```python
from build123d import *

# Parameters (mm, degrees)
SKETCH_1_W             = 42
SKETCH_1_H             = 45
SKETCH_1_R             = 12.5
EXTRUDE_1_DEPTH        = 35
SKETCH_3_W             = 24
SKETCH_3_H             = 37
CUT_EXTRUDE_1_DEPTH    = 71.809603868
HOLE_WIZARD_M3_2_D     = 2.5
HOLE_WIZARD_M3_2_DEPTH = 6
HOLE_WIZARD_M3_2_TIP   = 0.751075774
HOLE_WIZARD_M3_4_D     = 2.5
HOLE_WIZARD_M3_4_DEPTH = 6
HOLE_WIZARD_M3_4_TIP   = 0.751075774
SKETCH_18_W            = 28
SKETCH_18_H            = 20
CUT_EXTRUDE_8_DEPTH    = 71.809603868
SKETCH_13_R            = 2
CUT_EXTRUDE_10_DEPTH   = 71.809603868
FILLET_3_DEPTH         = 42
FILLET_7_R             = 2
CUT_EXTRUDE_9_REACH    = 72.81
SKETCH_12_R            = 13
SKETCH_12_R_2          = 12.5
SKETCH_12_R_3          = 2.5


with BuildPart() as part:
    # 草图1 → 凸台-拉伸1 (new body)
    with BuildSketch(Plane.XY):
        with Locations((21, 22.5)):
            Rectangle(SKETCH_1_W, SKETCH_1_H)
        with Locations((21, 22.5)):
            Circle(SKETCH_1_R, mode=Mode.SUBTRACT)
    extrude(amount=EXTRUDE_1_DEPTH)

    # 草图3 → 切除-拉伸1 (cut, through all)
    with BuildSketch(Plane.ZY):
        with Locations((20, 22.5)):
            Rectangle(SKETCH_3_W, SKETCH_3_H)
    extrude(amount=-CUT_EXTRUDE_1_DEPTH, mode=Mode.SUBTRACT)

    # M3 螺纹孔2
    with Locations(Plane(origin=(3.5, 45, 5), x_dir=(0, 0, 1), z_dir=(0, 1, 0))):
        with Locations((0, 0), (0, 35), (22, 35), (22, 0)):
            Hole(HOLE_WIZARD_M3_2_D / 2, depth=HOLE_WIZARD_M3_2_DEPTH)
            with Locations((0, 0, -(HOLE_WIZARD_M3_2_DEPTH + HOLE_WIZARD_M3_2_TIP / 2))):  # 118° drill point
                Cone(0, HOLE_WIZARD_M3_2_D / 2, HOLE_WIZARD_M3_2_TIP, mode=Mode.SUBTRACT)

    # M3 螺纹孔4
    with Locations(Plane(origin=(3.5, 0, 5), x_dir=(0, 0, -1), z_dir=(0, -1, 0))):
        with Locations((0, 0), (-22, 0), (-22, 35), (0, 35)):
            Hole(HOLE_WIZARD_M3_4_D / 2, depth=HOLE_WIZARD_M3_4_DEPTH)
            with Locations((0, 0, -(HOLE_WIZARD_M3_4_DEPTH + HOLE_WIZARD_M3_4_TIP / 2))):  # 118° drill point
                Cone(0, HOLE_WIZARD_M3_4_D / 2, HOLE_WIZARD_M3_4_TIP, mode=Mode.SUBTRACT)

    # 草图18 → 切除-拉伸8 (cut, through all)
    with BuildSketch(Plane(origin=(0, 45, 0), x_dir=(1, 0, 0), z_dir=(0, 1, 0))):
        with Locations((21, -20)):
            Rectangle(SKETCH_18_W, SKETCH_18_H)
    extrude(amount=-CUT_EXTRUDE_8_DEPTH, mode=Mode.SUBTRACT)

    # 草图13 → 切除-拉伸10 (cut, through all)
    with BuildSketch(Plane.XY.offset(35)):
        with Locations((33.727922061, 9.772077939)):
            Circle(SKETCH_13_R)
        with Locations((33.727922061, 35.227922061)):
            Circle(SKETCH_13_R)
        with Locations((8.272077939, 35.227922061)):
            Circle(SKETCH_13_R)
        with Locations((8.272077939, 9.772077939)):
            Circle(SKETCH_13_R)
    extrude(amount=-CUT_EXTRUDE_10_DEPTH, mode=Mode.SUBTRACT)

    # 圆角3: read off the stored shape, not the designer's step
    # 圆角3 outline → 圆角3 (add)
    with BuildSketch(Plane.YZ):
        with BuildLine():
            ThreePointArc((41, 10), (40.414213562, 8.585786438), (39, 8))
            Line((39, 8), (41, 8))
            Line((41, 8), (41, 10))
        make_face()
        with BuildLine():
            Line((4, 8), (6, 8))
            ThreePointArc((6, 8), (4.585786438, 8.585786438), (4, 10))
            Line((4, 10), (4, 8))
        make_face()
        with BuildLine():
            ThreePointArc((39, 32), (40.414213562, 31.414213562), (41, 30))
            Line((41, 30), (41, 32))
            Line((41, 32), (39, 32))
        make_face()
        with BuildLine():
            Line((4, 32), (4, 30))
            ThreePointArc((4, 30), (4.585786438, 31.414213562), (6, 32))
            Line((6, 32), (4, 32))
        make_face()
    extrude(amount=FILLET_3_DEPTH)

    # 圆角7
    fillet_7_edges = [part.edges().sort_by_distance(p)[0] for p in [
        (35, 2, 10),
        (35, 43, 10),
        (35, 2, 30),
        (35, 43, 30),
        (7, 2, 30),
        (7, 43, 30),
        (7, 2, 10),
        (7, 43, 10),
    ]]
    fillet(fillet_7_edges, radius=FILLET_7_R)

    # 草图12 → 切除-拉伸9 (cut, up to next)
    with BuildSketch(Plane(origin=(0, 0, 0), x_dir=(-1, 0, 0), z_dir=(0, 0, -1)), mode=Mode.PRIVATE) as cut_extrude_9_sk1:
        with Locations((-21, 22.5)):
            Circle(SKETCH_12_R)
        with Locations(Location((-21, 22.5, 0), (0, 0, 180))):
            Circle(SKETCH_12_R_2, mode=Mode.SUBTRACT)
    cut_extrude_9_tool1 = extrude(cut_extrude_9_sk1.sketch, amount=-CUT_EXTRUDE_9_REACH, mode=Mode.PRIVATE) & part.part
    # 草图12 → 切除-拉伸9 (cut, up to next)
    with BuildSketch(Plane(origin=(0, 0, 0), x_dir=(-1, 0, 0), z_dir=(0, 0, -1)), mode=Mode.PRIVATE) as cut_extrude_9_sk2:
        with Locations((-8.272077939, 35.227922061)):
            Circle(SKETCH_12_R_3)
    cut_extrude_9_tool2 = extrude(cut_extrude_9_sk2.sketch, amount=-CUT_EXTRUDE_9_REACH, mode=Mode.PRIVATE) & part.part
    # 草图12 → 切除-拉伸9 (cut, up to next)
    with BuildSketch(Plane(origin=(0, 0, 0), x_dir=(-1, 0, 0), z_dir=(0, 0, -1)), mode=Mode.PRIVATE) as cut_extrude_9_sk3:
        with Locations((-8.272077939, 9.772077939)):
            Circle(SKETCH_12_R_3)
    cut_extrude_9_tool3 = extrude(cut_extrude_9_sk3.sketch, amount=-CUT_EXTRUDE_9_REACH, mode=Mode.PRIVATE) & part.part
    # 草图12 → 切除-拉伸9 (cut, up to next)
    with BuildSketch(Plane(origin=(0, 0, 0), x_dir=(-1, 0, 0), z_dir=(0, 0, -1)), mode=Mode.PRIVATE) as cut_extrude_9_sk4:
        with Locations((-33.727922061, 9.772077939)):
            Circle(SKETCH_12_R_3)
    cut_extrude_9_tool4 = extrude(cut_extrude_9_sk4.sketch, amount=-CUT_EXTRUDE_9_REACH, mode=Mode.PRIVATE) & part.part
    # 草图12 → 切除-拉伸9 (cut, up to next)
    with BuildSketch(Plane(origin=(0, 0, 0), x_dir=(-1, 0, 0), z_dir=(0, 0, -1)), mode=Mode.PRIVATE) as cut_extrude_9_sk5:
        with Locations((-33.727922061, 35.227922061)):
            Circle(SKETCH_12_R_3)
    cut_extrude_9_tool5 = extrude(cut_extrude_9_sk5.sketch, amount=-CUT_EXTRUDE_9_REACH, mode=Mode.PRIVATE) & part.part
    add(cut_extrude_9_tool1.solids().sort_by_distance((33.632304, 22.5, 0))[0], mode=Mode.SUBTRACT)
    add(cut_extrude_9_tool2.solids().sort_by_distance((8.272078, 35.227922, 0))[0], mode=Mode.SUBTRACT)
    add(cut_extrude_9_tool3.solids().sort_by_distance((8.272078, 9.772078, 0))[0], mode=Mode.SUBTRACT)
    add(cut_extrude_9_tool4.solids().sort_by_distance((33.727922, 9.772078, 0))[0], mode=Mode.SUBTRACT)
    add(cut_extrude_9_tool5.solids().sort_by_distance((33.727922, 35.227922, 0))[0], mode=Mode.SUBTRACT)


solid = part.part
```
Source: CAD feature listing. Evaluate the final solid. Frame: model axes, mm. A direction names the side the tool comes from. Give positions to 0.01 mm unless a question says otherwise; leave off trailing zeros. Order: outer loops, then holes, each group sorted by start corner. A loop starts at its lowest first (then second) coordinate and runs counter-clockwise, first axis right, second up.
(1) Section query D-D (z = 17). Return the cut outline in (x, y).
(2) Material intervals for line 1 along X through (y, z) = (2, 27); line 2 along Y through (x, z) = (3, 23); line 3 along Z through (x, y) = (12, 3), sorted ascending.
(3) Section query B-B (x = 21). Return the cut outline in (y, z).
(4) Contact query for flat-ended pins moving along their axis: P1, Ø10, axis at x = 37.5, z = 12, coming from the -Y side; P2, Ø2, axis at x = 3.5, z = 5, coming from the -Y side. Output: stop coordinate, or through.
(5) Section query C-C (y = 22.5). Return the cut outline in (x, z), plus the area to 3 significant figures.
(6) Pull-direction query (X, two-part tool) for faces 5 (the face through (8.6, 12.25, 3.94)), 6 (the face through (20.71, 40.43, 8.6)); classes: +X half, -X half, draft (parallel to the pull), parting line (faces both ways), or undercut.
(7) Section query A-A (z = 27). State how many separate pieces and enclosed holes the cut face has, plus the area to 3 significant figures.
(8) Access query for faces 1 (the face through (37.391, 3.042, 5.577)), 2 (the face through (7.57, 42.97, 29.4)), 3 (the face through (20.71, 4.6, 8.57)), 4 (the face through (31.343, 10.523, 3.944)). Directions: +Z, -Z, +X, -X, +Y, -Y. A direction counts if a zero-diameter tool reaches every point of the face in a straight line with its end or side. Return the directions, or none.
Outcome:
1. outline: (0, 0) - (7, 0) - (7, 4) - (0, 4) - close; (0, 41) - (7, 41) - (7, 45) - (0, 45) - close; (35, 0) - (42, 0) - (42, 4) - (35, 4) - close; (35, 41) - (42, 41) - (42, 45) - (35, 45) - close
2. line 1: x = 0 to 2.25, 4.75 to 7, 35 to 37.25, 39.75 to 42
2. line 2: y = 0 to 4, 41 to 45
2. line 3: z = 0 to 10, 30 to 35
3. outline: (0, 0) - (9.5, 0) - (9.5, 8) - (6, 8) arc R2 cw to (4, 10) - (0, 10) - close; (0, 30) - (4, 30) arc R2 cw to (6, 32) - (10, 32) - (10, 35) - (0, 35) - close; (35, 32) - (39, 32) arc R2 cw to (41, 30) - (45, 30) - (45, 35) - (35, 35) - close; (35.5, 0) - (45, 0) - (45, 10) - (41, 10) arc R2 cw to (39, 8) - (35.5, 8) - close
4. P1: stops at y = 0
4. P2: stops at y = 6.15
5. outline: (0, 0) - (8, 0) - (8, 8) - (0, 8) - close; (0, 32) - (8.5, 32) - (8.5, 35) - (0, 35) - close; (33.5, 32) - (42, 32) - (42, 35) - (33.5, 35) - close; (34, 0) - (42, 0) - (42, 8) - (34, 8) - close
5. area: 179 mm2
6. face 5: undercut
6. face 6: draft
7. separate pieces: 8
7. enclosed holes: 0
7. area: 72.0 mm2
8. face 1: -Y
8. face 2: +Y, -Y
8. face 3: +X, -X
8. face 4: -Z
